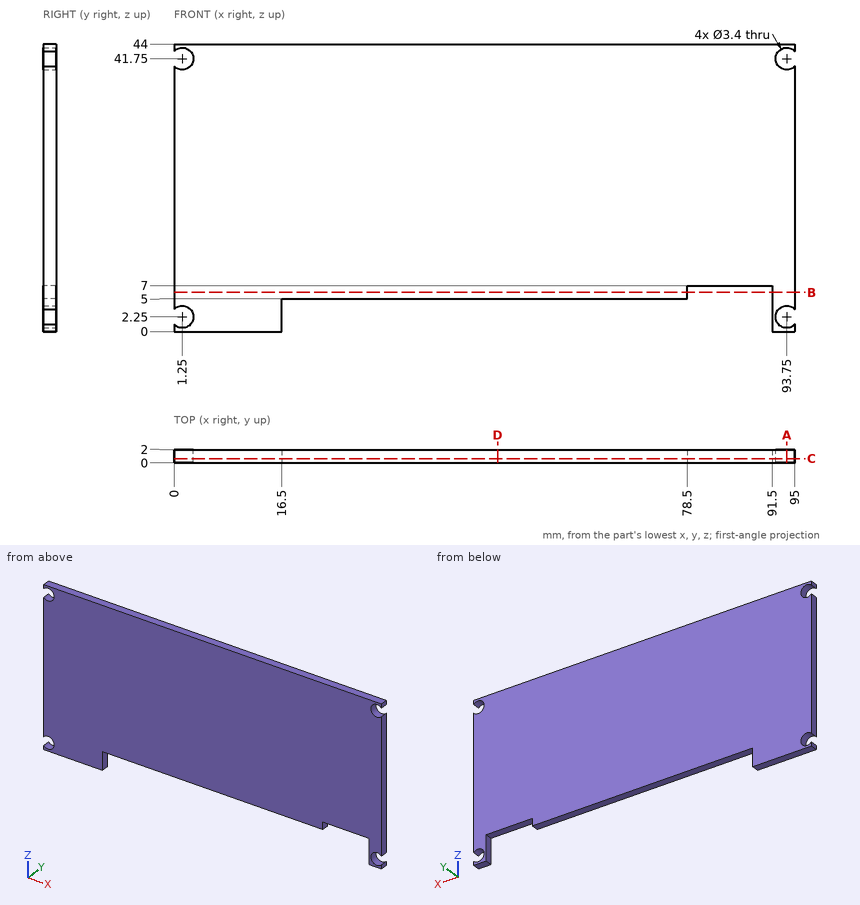
Answer from the drawing. Dimensions are ordinates in mm from the lowest x, y and z of the part. Give positions to 0.01 mm unless a question says otherwise; leave off trailing zeros. Order: outer loops, then holes, each group sorted by start corner. A loop starts at its lowest first (then second) coordinate and runs counter-clockwise, first axis right, second up.
(1) Find section D-D (x = 49.5). Give the vertices of the cut face in (y, z).
(2) Given pin 1 (1 mm diameter, centred on y = 1, z = 2, fed in from +X); pin 2 (0.6 mm diameter, centred on x = 62.5, y = 1, fed in from -Z); pin 3 (1 mm diameter, centred on x = 83.5, y = 1, fed in from -Z), each flat-ended and moving along its own axis, determine where each tip first touches the part or whether it passes through.
(3) Find section C-C (y = 0.6). Give the vertices of the cut face in (x, z).
(4) Straight lines are drawn through the part: L1, parallel to Z at x = 93.75, y = 1.05; L2, parallel to Z at x = 45, y = 0.2; L3, parallel to X at y = 0.8, z = 41.75. For each, find the intervals that lie inside material, in ascending order.
(5) Find section A-A (x = 93.75). Give the vertices of the cut face in (y, z).
(6) Find section B-B (z = 6). Give the vertices of the cut face in (x, y).
Result sheet:
1. outline: (0, 5) - (2, 5) - (2, 44) - (0, 44) - close
2. pin 1: stops at x = 92.22
2. pin 2: stops at z = 5
2. pin 3: stops at z = 7
3. outline: (0, 0) - (16.5, 0) - (16.5, 5) - (78.5, 5) - (78.5, 7) - (91.5, 7) - (91.5, 0) - (95, 0) - (95, 1.1) arc R1.7 cw (long way) to (95, 3.4) - (95, 40.6) arc R1.7 cw (long way) to (95, 42.9) - (95, 44) - (0, 44) - (0, 42.9) arc R1.7 cw (long way) to (0, 40.6) - (0, 3.4) arc R1.7 cw (long way) to (0, 1.1) - close
4. L1: z = 0 to 0.55, 3.95 to 40.05, 43.45 to 44
4. L2: z = 5 to 44
4. L3: x = 2.95 to 92.05
5. outline: (0, 0) - (2, 0) - (2, 0.55) - (0, 0.55) - close; (0, 3.95) - (2, 3.95) - (2, 40.05) - (0, 40.05) - close; (0, 43.45) - (2, 43.45) - (2, 44) - (0, 44) - close
6. outline: (0, 0) - (78.5, 0) - (78.5, 2) - (0, 2) - close; (91.5, 0) - (95, 0) - (95, 2) - (91.5, 2) - close
